Can you work these out from the model? Positions are in its coordinate system, mm. A direction names the side the tool comes from. Coordinates: 2 decimals unless noted, no trailing zeros. Loops run counter-clockwise (first coordinate to the right, second up) from the corner with the lowest first, then second, coordinate; pieces in that order, holes last. Notation, with made-up numbers: M -6.5,24.25 L 3.5,24.25 A24 cw 3.5,53.25 Z; hole C 87.25,-8 d8. An arc over 180 degrees is marked long. Answer as a JSON object with one key per item and string values. Group by question number.
Item 1: Suppose I cut it at B-B (z = 5.5). Write out the boundary of the cut face in (x, y), then the cut area to 3 significant figures.
Item 2: Suppose I cut it at A-A (x = 0). Write out the boundary of the cut face in (y, z), then the cut area to 3 significant figures.
Item 3: If I drill on line 1 (X direction, y = -0.25, z = 4.5); line 2 (Y direction, x = -2, z = 2), over which ranges is the centre line in solid material (lowest first)?
Item 4: Suppose I cut it at C-C (z = 7.5). Write out the boundary of the cut face in (x, y), then the cut area to 3 significant figures.
Item 5: Which directions (+Z, -Z, +X, -X, +Y, -Y) give clear straight access to the entire face, cutting with the end or side of a thin tool? Please do faces 1 (the flat face through (2.4, -6.1, 8)), 2 (the flat face through (-5, 3, 2.41)).
Item 6: I'm going to push flat-ended pins straight in: pin 1 Ø1 at (x, z) = (1, 6.5) entering from -Y; pin 2 Ø1.5 at (x, z) = (-3.5, 1.5) entering from -Y; pin 3 Ø10 at (x, y) = (0, 0) entering from +Z (3 decimals); pin 4 Ø2 at (x, z) = (-2, 4) entering from -Y. Where does each tip first touch, or does it pass through?
Item 7: We'd pull the mould along X, two halves only. Please class faces 3 (the cylindrical face through (-1.172, 8.923, 3.972)), 4 (the flat face through (1.7, -5.4, 0)), 5 (the cylindrical face through (-1.38, -6.2, 5.17)), 6 (the cylindrical face through (-1.19, -5.37, 1.19)): +X half, -X half, draft (parallel to the pull), parting line (faces both ways), or undercut.
```python
from build123d import *

# Parameters (mm, degrees)
F0_R     = 6.35
F0_R_2   = 5.5
F1_DEPTH = 2.41
F0_R_3   = 9
F2_DEPTH = 8
F3_SIZE2 = 0.72794
F3_SIZE  = 2
F4_SIZE2 = 0.72794
F4_SIZE  = 2


with BuildPart() as f1:
    # F0 (on Top) → F1 (new body)
    with BuildSketch(Plane.XY):
        Circle(F0_R)
        Circle(F0_R_2, mode=Mode.SUBTRACT)
    extrude(amount=F1_DEPTH)

    # F0 (on Top) → F2 (join)
    with BuildSketch(Plane.XY):
        Circle(F0_R_3)
        Circle(F0_R, mode=Mode.SUBTRACT)
    extrude(amount=F2_DEPTH)

    # F3
    f3_edges = [f1.edges().sort_by_distance(p)[0] for p in [
        (-9, 0, 0),
    ]]
    chamfer(f3_edges, length=F3_SIZE, length2=F3_SIZE2)

    # F4
    f4_edges = [f1.edges().sort_by_distance(p)[0] for p in [
        (-9, 0, 8),
    ]]
    chamfer(f4_edges, length=F4_SIZE, length2=F4_SIZE2)


solid = f1.part
```
From the geometry:
{
 "1": {"outline": "C 0,0 d18; hole C 0,0 d12.7", "area": "128 mm2"},
 "2": {"outline": "M -9,2 L -8.27,0 L -5.5,0 L -5.5,2.41 L -6.35,2.41 L -6.35,8 L -8.27,8 L -9,6 Z; M 5.5,0 L 8.27,0 L 9,2 L 9,6 L 8.27,8 L 6.35,8 L 6.35,2.41 L 5.5,2.41 Z", "area": "43.6 mm2"},
 "3": {"line 1": "-9 to -6.35, 6.35 to 9", "line 2": "-8.77 to -5.12, 5.12 to 8.77"},
 "4": {"outline": "C 0,0 d16.91; hole C 0,0 d12.7", "area": "97.9 mm2"},
 "5": {"face 1": "+Z, +X, -X, +Y, -Y", "face 2": "+Z"},
 "6": {"pin 1": "y = -8.95", "pin 2": "y = -8.51", "pin 3": "through", "pin 4": "y = -8.94"},
 "7": {"face 3": "parting line", "face 4": "draft", "face 5": "undercut", "face 6": "undercut"}
}
